Check sheet for the modelled part. Datum: model origin and axes. Units: mm. Face numbers are marked on the shaded views. A direction names the side the tool comes from. Round coordinates to 2 decimals unless told otherwise and drop trailing zeros. Write each loop counter-clockwise with the first axis right and the second up, starting at its lowest first coordinate (ties: lowest second). Pieces come first, ordered by that corner, then holes.
from build123d import *

# Parameters (mm, degrees)
F0_R      = 5.5
F1_DEPTH  = 15.5
F2_R      = 1.5
F3_DEPTH  = 9
F5_R      = 1.25
F6_DEPTH  = 6
F4_R      = 1.5
F7_DEPTH  = 5.1
F9_DEPTH  = 25.4
F11_ANGLE = 180
F13_ANGLE = -90
F15_ANGLE = 90


# Not quite as in the source:
# - a feature names something its author has since deleted; it is built from what else it names


with BuildPart() as f1:
    # F0 (on Top) → F1 (new body)
    with BuildSketch(Plane.XY):
        Circle(F0_R)
    extrude(amount=F1_DEPTH)

    # F2 (on face) → F3 (cut)
    with BuildSketch(Plane(origin=(0, 0, 0), x_dir=(1, 0, 0), z_dir=(0, 0, -1))):
        Circle(F2_R)
    extrude(amount=-F3_DEPTH, mode=Mode.SUBTRACT)

    # F5 (on face) → F6 (cut)
    with BuildSketch(Plane.XY.offset(15.5)):
        Circle(F5_R)
    extrude(amount=-F6_DEPTH, mode=Mode.SUBTRACT)

    # F4 (on face) → F7 (cut)
    with BuildSketch(Plane(origin=(0, 0, 0), x_dir=(1, 0, 0), z_dir=(0, 0, -1))):
        Polygon((2, 3.5), (-2, 3.5), (-4.0207259422, 0), (-2, -3.5), (2, -3.5), (4.0207259422, 0), align=None)
        Circle(F4_R, mode=Mode.SUBTRACT)
    extrude(amount=-F7_DEPTH, mode=Mode.SUBTRACT)

    # F8 (on face) → F9 (cut)
    with BuildSketch(Plane.XZ.offset(-3.5)):
        with BuildLine():
            ThreePointArc((1.75, 2.55), (-1.2374368671, 3.7874368671), (0, 0.8))
            ThreePointArc((0, 0.8), (1.2374368671, 1.3125631329), (1.75, 2.55))
        make_face()
    extrude(amount=-F9_DEPTH, mode=Mode.SUBTRACT)


with BuildPart() as f1_1:
    # F11: moved
    add(f1.part.rotate(Axis((9.4123384915, 0, 0), (1, 0, 0)), F11_ANGLE))


with BuildPart() as f1_2:
    # F13: moved
    add(f1_1.part.rotate(Axis((-2.3788576946, 0, 0), (-1, 0, 0)), F13_ANGLE))


with BuildPart() as f1_3:
    # F15: moved
    add(f1_2.part.rotate(Axis((0, 5.9970328584, 0), (0, -1, 0)), F15_ANGLE))


solid = f1_3.part
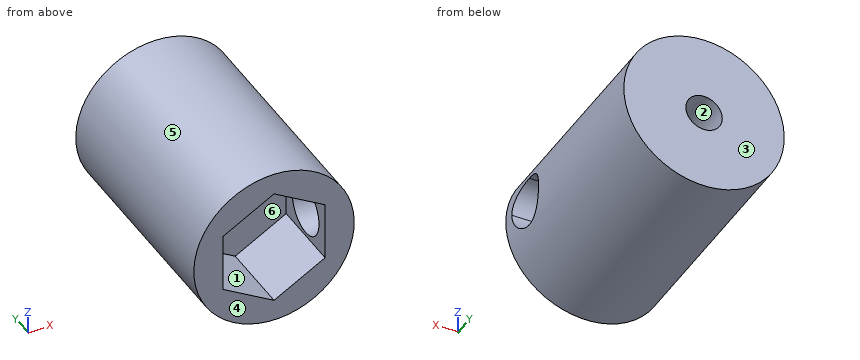
1. Set-up check for the marked faces 1, 2 and 3: record each of +Z, -Z, +X, -X, +Y, -Y from which the full face is reachable in a straight line by a thin tool's end or side.
2. Sectioned sample at C-C, the plane x = 4. Enter the section's corners in (y, z), plus the area to 3 significant figures.
3. Sectioned sample at D-D, the plane y = 2.75. Enter the section's corners in (x, z).
4. Release check for a two-part mould opening along Z. For the marked faces 4, 5 and 6 record: released by +Z, released by -Z, zero draft, split by the parting line, or undercut.
5. Sectioned sample at B-B, the plane y = 10. Enter the section's corners in (x, z).
6. Sectioned sample at A-A, the plane x = 1.75. Enter the section's corners in (y, z), plus the area to 3 significant figures.
7. Go/stop test with flat-tipped pins: pin 1 (4 mm diameter, centred on x = 0, z = 0, fed in from -Y); pin 2 (3 mm diameter, centred on x = -2, y = 3, fed in from +Z); pin 3 (5 mm diameter, centred on y = 9.5, z = -3, fed in from +X). Record where each tip stops, or that it passes through.
8. Scan lines: line 1 along Y through (x, z) = (4.35, 0); line 2 along X through (y, z) = (11.4, 0); line 3 along X through (y, z) = (6.5, 0). Record each from-to range of solid material in increasing order.
Computed values:
1. face 1: -Y
1. face 2: +Y
1. face 3: +Z, -Z, +X, -X, +Y
2. outline: (0, -3.77) - (15.5, -3.77) - (15.5, 3.77) - (0, 3.77) - close; hole circle Ø3.5 at (2.55, 0)
2. area: 107 mm2
3. outline: (-3.5, -2) - (-3.5, 2) - (0, 4.02) - (3.5, 2) - (3.5, 1.74) - (5.22, 1.74) arc R5.5 ccw (long way) to (5.22, -1.74) - (3.5, -1.74) - (3.5, -2) - (0, -4.02) - close
4. face 4: zero draft
4. face 5: split by the parting line
4. face 6: undercut
5. outline: circle Ø11 at (0, 0); hole circle Ø2.5 at (0, 0)
6. outline: (0, -5.21) - (15.5, -5.21) - (15.5, 5.21) - (0, 5.21) - (0, 3.01) - (5.1, 3.01) - (5.1, -3.01) - (0, -3.01) - close
6. area: 131 mm2
7. pin 1: stops at y = 5.1
7. pin 2: stops at z = 5.48
7. pin 3: stops at x = 5.48
8. line 1: y = 0 to 0.8, 4.3 to 15.5
8. line 2: x = -5.5 to -1.25, 1.25 to 5.5
8. line 3: x = -5.5 to -1.5, 1.5 to 5.5
